Autodesk Fusion 360 part; units mm, degrees
sketch "base_sketch" plane through (0, 0, 0) normal (0, 1, 0) x (1, 0, 0) in component "bed"
  line L0 (176, -176) -> (-176, -176)
  line L1 (-176, -176) -> (-176, 176)
  line L2 (-176, 176) -> (176, 176)
  line L3 (176, 176) -> (176, -176)
  line L4 (176, -176) -> (-176, 176) construction
  line L5 (-176, -176) -> (176, 176) construction
  circle A0 centre (0, 0) radius 4.5
  line L6 (-176, -176) -> (-160, -176)
  line L7 (-160, -176) -> (-160, -158)
  line L8 (-160, -158) -> (-176, -158)
  line L9 (-176, -158) -> (-176, -176)
  line L10 (176, -176) -> (160, -176)
  line L11 (160, -176) -> (160, -158)
  line L12 (160, -158) -> (176, -158)
  line L13 (176, -158) -> (176, -176)
  line L14 (-50, 176) -> (50, 176)
  line L15 (50, 176) -> (50, 161)
  line L16 (50, 161) -> (-50, 161)
  line L17 (-50, 161) -> (-50, 176)
  line L18 (0, 176) -> (0, -176) construction
  dimension "d18" = 352
  dimension "d19" = 352
  dimension "d20" = 9
  dimension "d21" = 16
  dimension "d22" = 18
  dimension "d23" = 16
  dimension "d24" = 18
  dimension "d26" = 15
  dimension "d30" = 50
extrude "Extrude1" add sketch "base_sketch" along normal blind 2 contours L0 L1 L2 L3 L7 L8 L11 L12 L15 L16 L17 in component "bed"
fillet "Fillet1" radius 5 2 edges at (160, 1, 158) (-160, 1, 158) in component "bed"
fillet "Fillet2" radius 4 2 edges at (-50, 1, -161) (50, 1, -161) in component "bed"
fillet "Fillet3" radius 2 8 edges at (-176, 1, -176) (50, 1, -176) (-50, 1, -176) (176, 1, -176) (176, 1, 158) (160, 1, 176) (-160, 1, 176) (-176, 1, 158) in component "bed"
sketch "export_dxf" plane through (0, 2, 0) normal (0, 1, 0) x (-1, 0, 0) in component "bed"
  arc A0 (176, 156) -> (174, 158) centre (174, 156) ccw
  line L0 (174, 158) -> (165, 158)
  arc A1 (160, 163) -> (165, 158) centre (165, 163) ccw
  line L1 (160, 163) -> (160, 174)
  arc A2 (160, 174) -> (158, 176) centre (158, 174) ccw
  line L2 (158, 176) -> (-158, 176)
  arc A3 (-158, 176) -> (-160, 174) centre (-158, 174) ccw
  line L3 (-160, 174) -> (-160, 163)
  arc A4 (-165, 158) -> (-160, 163) centre (-165, 163) ccw
  line L4 (-165, 158) -> (-174, 158)
  arc A5 (-174, 158) -> (-176, 156) centre (-174, 156) ccw
  line L5 (-176, 156) -> (-176, -174)
  arc A6 (-176, -174) -> (-174, -176) centre (-174, -174) ccw
  line L6 (-174, -176) -> (-52, -176)
  arc A7 (-52, -176) -> (-50, -174) centre (-52, -174) ccw
  line L7 (-50, -174) -> (-50, -165)
  arc A8 (-46, -161) -> (-50, -165) centre (-46, -165) ccw
  line L8 (-46, -161) -> (46, -161)
  arc A9 (50, -165) -> (46, -161) centre (46, -165) ccw
  line L9 (50, -165) -> (50, -174)
  arc A10 (50, -174) -> (52, -176) centre (52, -174) ccw
  line L10 (52, -176) -> (174, -176)
  arc A11 (174, -176) -> (176, -174) centre (174, -174) ccw
  line L11 (176, -174) -> (176, 156)
  circle A12 centre (0, 0) radius 4.5
component "bed" placed x (1, 0, 0) y (0, 1, 0) z (0, 0, 1) at (0, 0, 0)
Geometry: final body of the model. Coordinates: model frame, mm. Coordinates: 2 decimals unless noted, no trailing zeros. Write each loop counter-clockwise with the first axis right and the second up, starting at its lowest first coordinate (ties: lowest second). Pieces come first, ordered by that corner, then holes. Notation, with made-up numbers: M 35,-14.75 L 86,-14.75 A20 ccw 86,10.25 Z; hole C 7,66.5 d6. An arc over 180 degrees is marked long. Use CSV: the item, a comma, the result in double quotes. Start each with the question number.
1. Cut plane B-B on z = 0. Return the cut outline in (x, y), plus the area to 3 significant figures.
2. Cut plane C-C on x = 0. Return the cut outline in (y, z).
3. Ray query, probe 1 along X at (y, z) = (1.25, 0); probe 2 along Z at (x, y) = (0, 0.5); probe 3 along Z at (x, y) = (-5, 1.15). Return the intervals inside material, ascending.
4. Mould query, pull axis Z, two halves, no side actions, for faces 1 (the face through (-0.59, 0.99, 4.46)), 2 (the face through (-42, 2, -2)). Classes: pulls with the +Z half, pulls with the -Z half, needs draft (parallel to the pull), parting line crosses it, or undercut.
5. Cut plane A-A on y = 0.55. Return the cut outline in (x, z).
6. First-contact query: P1, Ø1, axis at y = 1.5, z = 167, coming from the -X side; P2, Ø1, axis at y = 1, z = 168, coming from the +X side; P3, Ø0.6, axis at x = 171.5, y = 1, coming from the +Z side. Flat tips, straight axial feed; report the tip coordinate or a pass-through.
Entries:
1,outline,"M -176,0 L -4.5,0 L -4.5,2 L -176,2 Z; M 4.5,0 L 176,0 L 176,2 L 4.5,2 Z"
1,area,"686 mm²"
2,outline,"M 0,-161 L 2,-161 L 2,-4.5 L 0,-4.5 Z; M 0,4.5 L 2,4.5 L 2,176 L 0,176 Z"
3,probe 1,"-176 to -4.5, 4.5 to 176"
3,probe 2,"-161 to -4.5, 4.5 to 176"
3,probe 3,"-161 to 176"
4,face 1,"undercut"
4,face 2,"needs draft"
5,outline,"M -176,-174 A2 ccw -174,-176 L -52,-176 A2 ccw -50,-174 L -50,-165 A4 cw -46,-161 L 46,-161 A4 cw 50,-165 L 50,-174 A2 ccw 52,-176 L 174,-176 A2 ccw 176,-174 L 176,156 A2 ccw 174,158 L 165,158 A5 cw 160,163 L 160,174 A2 ccw 158,176 L -158,176 A2 ccw -160,174 L -160,163 A5 cw -165,158 L -174,158 A2 ccw -176,156 Z; hole C 0,0 d9"
6,P1,"x = -160"
6,P2,"x = 160"
6,P3,"z = 158"
